Geometry: final body of the model. Coordinates: model frame, mm. A direction names the side the tool comes from. Round coordinates to 2 decimals unless told otherwise and drop trailing zeros. Write each loop counter-clockwise with the first axis right and the second up, starting at its lowest first coordinate (ties: lowest second). Pieces come first, ordered by that corner, then holes. Notation, with made-up numbers: (-11.5, 41) -> (11.5, 41) arc R17 ccw to (11.5, 65) -> close; hole circle Ø6 at (7.25, -27). An arc over 180 degrees is marked (long way). One line per item, written item: value. Start each with the question number.
from build123d import *

# Parameters (mm, degrees)
EXTRUDE_2_DEPTH      = 11
EXTRUDE_2_DEPTH_BACK = 11
EXTRUDE_3_DEPTH      = 1
SKETCH_9_R           = 4
CUT_EXTRUDE_5_DEPTH  = 15
CUT_EXTRUDE_6_DEPTH  = 15
CHAMFER_1_SIZE       = 5
CHAMFER_2_SIZE       = 5
SKETCH_11_R          = 4
SKETCH_11_W          = 30
SKETCH_11_H          = 22
EXTRUDE_5_DEPTH      = 2


with BuildPart() as part:
    # Эскиз3 → Бобышка-Вытянуть2 (new, two sides: drawn at the far end of the back side and taken through both)
    with BuildSketch(Plane.XY.offset(-EXTRUDE_2_DEPTH_BACK)):
        with BuildLine():
            ThreePointArc((15, 95), (0, 80), (-15, 95))
            Line((-15, 95), (-27.5, 95))
            Line((-27.5, 95), (-27.5, 80))
            Line((-27.5, 80), (-15, 80))
            Line((-15, 80), (-15, 75))
            ThreePointArc((-15, 75), (0, 70), (15, 75))
            Line((15, 75), (15, 80))
            Line((15, 80), (27.5, 80))
            Line((27.5, 80), (27.5, 95))
            Line((27.5, 95), (15, 95))
        make_face()
    extrude(amount=EXTRUDE_2_DEPTH + EXTRUDE_2_DEPTH_BACK)

    # Эскиз5 → Бобышка-Вытянуть3 (add)
    with BuildSketch(Plane.XY.offset(11)):
        with BuildLine():
            Line((-19, 95), (-15, 95))
            ThreePointArc((-15, 95), (0, 80), (15, 95))
            Line((15, 95), (19, 95))
            ThreePointArc((19, 95), (0, 76), (-19, 95))
        make_face()
    extrude_3 = extrude(amount=EXTRUDE_3_DEPTH)

    # Зеркальное отражение1: Бобышка-Вытянуть3 across plane
    add(extrude_3.mirror(Plane.XY))

    # Эскиз9 → Вырез-Вытянуть5 (cut)
    with BuildSketch(Plane(origin=(0, 95, 0), x_dir=(1, 0, 0), z_dir=(0, 1, 0))):
        with Locations(Location((21, 0, 0), (0, 0, 270))):
            Circle(SKETCH_9_R)
        with Locations(Location((-21, 0, 0), (0, 0, 270))):
            Circle(SKETCH_9_R)
    extrude(amount=-CUT_EXTRUDE_5_DEPTH, mode=Mode.SUBTRACT)

    # Эскиз10 → Вырез-Вытянуть6 (cut)
    with BuildSketch(Plane.XZ.offset(-80)):
        with BuildLine():
            Line((27.5, -11), (27.5, 0))
            ThreePointArc((27.5, 0), (25.596194078, -4.596194078), (21, -6.5))
            Line((21, -6.5), (21, -11))
            Line((21, -11), (27.5, -11))
        make_face()
        with BuildLine():
            Line((21, 11), (21, 6.5))
            ThreePointArc((21, 6.5), (25.596194078, 4.596194078), (27.5, 0))
            Line((27.5, 0), (27.5, 11))
            Line((27.5, 11), (21, 11))
        make_face()
    cut_extrude_6 = extrude(amount=-CUT_EXTRUDE_6_DEPTH, mode=Mode.SUBTRACT)

    # Зеркальное отражение2: Вырез-Вытянуть6 across plane
    add(cut_extrude_6.mirror(Plane(origin=(0, 0, 0), x_dir=(0, 0, 1), z_dir=(1, 0, 0))), mode=Mode.SUBTRACT)

    # Фаска1
    # the kernel refuses this chamfer: 20, 5 mm, written as the material it takes off along each edge
    with BuildSketch(Plane(origin=(-15, 75, -36.862227042), x_dir=(0.9002602258420863, -0.4353521858986766, 0), z_dir=(0, 0, 1))) as chamfer_1_piece_1_section:
        with BuildLine():
            Line((9.593719339, 0), (-CHAMFER_1_SIZE * 0.435352185899, CHAMFER_1_SIZE * 0.900260225842))
            Line((-CHAMFER_1_SIZE * 0.435352185899, CHAMFER_1_SIZE * 0.900260225842), (0, 0))
            ThreePointArc((0, 0), (5.175297631, -0.461648225), (9.593719339, 0))
        make_face()
    chamfer_1_piece_1 = extrude(amount=73.724454084, mode=Mode.PRIVATE)
    chamfer_1_piece_1 = split(chamfer_1_piece_1, bisect_by=Plane(origin=(-15, 80, -36.862227042), z_dir=(0, -1, 0)), keep=Keep.TOP, mode=Mode.PRIVATE)
    add(chamfer_1_piece_1, mode=Mode.SUBTRACT)

    # Фаска2
    # the kernel refuses this chamfer: 20, 5 mm, written as the material it takes off along each edge
    with BuildSketch(Plane(origin=(15, 75, -36.862227042), x_dir=(-0.9002602258420859, -0.43535218589867725, 0), z_dir=(0, 0, 1))) as chamfer_2_piece_1:
        with BuildLine():
            Line((9.593719339, 0), (-CHAMFER_2_SIZE * 0.435352185899, -CHAMFER_2_SIZE * 0.900260225842))
            Line((-CHAMFER_2_SIZE * 0.435352185899, -CHAMFER_2_SIZE * 0.900260225842), (0, 0))
            ThreePointArc((0, 0), (5.175297631, 0.461648225), (9.593719339, 0))
        make_face()
    extrude(amount=73.724454084, mode=Mode.SUBTRACT)

    # Эскиз11 → Бобышка-Вытянуть5 (add)
    # profile 1 of 3: a face of its own
    with BuildSketch(Plane.XZ.offset(-80)):
        with BuildLine():
            Line((-15, 11), (-21, 11))
            Line((-21, 11), (-21, 6.5))
            ThreePointArc((-21, 6.5), (-27.5, 0), (-21, -6.5))
            Line((-21, -6.5), (-21, -11))
            Line((-21, -11), (-15, -11))
            Line((-15, -11), (-15, 11))
        make_face()
        with Locations(Location((-21, 0, 0), (0, 0, 90))):
            Circle(SKETCH_11_R, mode=Mode.SUBTRACT)
    # profile 2 of 3: a face of its own
    with BuildSketch(Plane.XZ.offset(-80)):
        with BuildLine():
            Line((21, -11), (21, -6.5))
            ThreePointArc((21, -6.5), (27.5, 0), (21, 6.5))
            Line((21, 6.5), (21, 11))
            Line((21, 11), (15, 11))
            Line((15, 11), (15, -11))
            Line((15, -11), (21, -11))
        make_face()
        with Locations(Location((21, 0, 0), (0, 0, 90))):
            Circle(SKETCH_11_R, mode=Mode.SUBTRACT)
    # profile 3 of 3: a face of its own
    with BuildSketch(Plane.XZ.offset(-80)):
        Rectangle(SKETCH_11_W, SKETCH_11_H)
    extrude(amount=EXTRUDE_5_DEPTH)


solid = part.part
(1) Section query D-D (y = 92). Output: boundary loops of the cut face in (x, z).
(2) Pull-direction query (X, two-part tool) for faces 1 (the face through (0, 80, 0)), 2 (the face through (0.418, 76.005, -11.493)), 3 (the face through (-17, 95, 3)); classes: pulls with the +X half, pulls with the -X half, needs draft (parallel to the pull), parting line crosses it, or undercut.
(3) Line query: probe 1 along X at (y, z) = (78.65, 0); probe 2 along X at (y, z) = (78.5, 3); probe 3 along X at (y, z) = (90.75, 0). Output: solid intervals per line, ascending.
(4) Pin query (flat end, axial travel): pin 1 (2 mm diameter, centred on x = 18.5, y = 88.5, fed in from -Z); pin 2 (2 mm diameter, centred on y = 78.5, z = -9, fed in from +X); pin 3 (3.5 mm diameter, centred on y = 85.5, z = -9.5, fed in from -X); pin 4 (1 mm diameter, centred on x = -21.5, z = -5, fed in from -Y). Return the tip coordinate at first contact, or that it passes through.
(5) Set-up query: faces 4 (the face through (0, 75, -11)), 5 (the face through (0, 75, 11)), 6 (the face through (-21, 87, 9)), 7 (the face through (-17, 78, -2)), 8 (the face through (-21, 87, -9)). Return all of +Z, -Z, +X, -X, +Y, -Y with unobstructed straight access to the full face (end or side cutting, diameter ignored); none if empty.
(6) Section query B-B (z = 3). Output: boundary loops of the cut face in (x, y).
(7) Section query C-C (x = 20). Output: boundary loops of the cut face in (y, z).
(8) Section query A-A (y = 88.25). Output: boundary loops of the cut face in (x, z), and give its area (3 significant figures).
Results list:
1. outline: (-21, -11) -> (-18.76, -11) -> (-18.76, -12) -> (-14.7, -12) -> (-14.7, 12) -> (-18.76, 12) -> (-18.76, 11) -> (-21, 11) -> (-21, 6.5) arc R6.5 ccw to (-21, -6.5) -> close; (14.7, -12) -> (18.76, -12) -> (18.76, -11) -> (21, -11) -> (21, -6.5) arc R6.5 ccw to (21, 6.5) -> (21, 11) -> (18.76, 11) -> (18.76, 12) -> (14.7, 12) -> close; hole circle Ø8 at (-21, 0); hole circle Ø8 at (21, 0)
2. face 1: undercut
2. face 2: parting line crosses it
2. face 3: needs draft
3. probe 1: x = -27.5 to -25, -17 to 17, 25 to 27.5
3. probe 2: x = -26.77 to -23.65, -18.35 to 18.35, 23.65 to 26.77
3. probe 3: x = -27.5 to -25, -17 to -14.39, 14.39 to 17, 25 to 27.5
4. pin 1: stops at z = -12
4. pin 2: stops at x = 21
4. pin 3: stops at x = -21
4. pin 4: stops at y = 78
5. face 4: -Z, -Y
5. face 5: +Z, -Y
5. face 6: +Z, -X, +Y, -Y
5. face 7: +Z, -Z, -X, -Y
5. face 8: -Z, -X, +Y, -Y
6. outline: (-26.77, 78) -> (-23.65, 78) -> (-23.65, 95) -> (-26.77, 95) -> close; (-18.35, 78) -> (-13.12, 78) -> (-6.36, 70.82) arc R25 ccw to (6.36, 70.82) -> (13.12, 78) -> (18.35, 78) -> (18.35, 95) -> (15, 95) arc R15 cw to (-15, 95) -> (-18.35, 95) -> close; (23.65, 78) -> (26.77, 78) -> (26.77, 95) -> (23.65, 95) -> close
7. outline: (78, -11) -> (95, -11) -> (95, -3.87) -> (78, -3.87) -> close; (78, 3.87) -> (95, 3.87) -> (95, 11) -> (78, 11) -> close
8. outline: (-21, -11) -> (-17.76, -11) -> (-17.76, -12) -> (-13.4, -12) -> (-13.4, 12) -> (-17.76, 12) -> (-17.76, 11) -> (-21, 11) -> (-21, 6.5) arc R6.5 ccw to (-21, -6.5) -> close; (13.4, -12) -> (17.76, -12) -> (17.76, -11) -> (21, -11) -> (21, -6.5) arc R6.5 ccw to (21, 6.5) -> (21, 11) -> (17.76, 11) -> (17.76, 12) -> (13.4, 12) -> close; hole circle Ø8 at (-21, 0); hole circle Ø8 at (21, 0)
8. area: 384 mm^2
